from build123d import *

# Parameters (mm, degrees)
F0_W     = 101.6
F0_H     = 101.6
F1_DEPTH = 38.1
F3_DEPTH = 101.601
F5_DEPTH = 101.601
F6_R     = 5.08


with BuildPart() as f1:
    # F0 (on Top) → F1 (new body)
    with BuildSketch(Plane.XY):
        with Locations((4.577692, -1.507951)):
            Rectangle(F0_W, F0_H)
    extrude(amount=F1_DEPTH)

    # F2 (on face) → F3 (cut, through all)
    with BuildSketch(Plane.XZ.offset(52.307951)):
        Polygon((10.344626, 38.1), (-1.188108, 38.1), (-8.121741, 19.05), (17.278259, 19.05), align=None)
    extrude(amount=-F3_DEPTH, mode=Mode.SUBTRACT)

    # F4 (on face) → F5 (cut, through all)
    with BuildSketch(Plane(origin=(-46.222308, 0, 0), x_dir=(0, -1, 0), z_dir=(-1, 0, 0))):
        Polygon((7.274885, 38.1), (-4.257849, 38.1), (-11.191482, 19.05), (14.208518, 19.05), align=None)
    extrude(amount=-F5_DEPTH, mode=Mode.SUBTRACT)

    # F6
    f6_edges = [f1.edges().sort_by_distance(p)[0] for p in [
        (32.861159, -52.307951, 38.1),
        (-23.705208, -52.307951, 38.1),
        (-46.222308, -29.791418, 38.1),
        (-46.222308, 26.774949, 38.1),
        (55.377692, 26.774949, 38.1),
        (55.377692, -29.791418, 38.1),
        (-23.705208, 49.292049, 38.1),
        (32.861159, 49.292049, 38.1),
        (-46.222308, -52.307951, 19.05),
        (55.377692, -52.307951, 19.05),
        (-46.222308, 49.292049, 19.05),
        (55.377692, 49.292049, 19.05),
    ]]
    fillet(f6_edges, radius=F6_R)


solid = f1.part
Part model, mm, in its own coordinate system. A direction names the side the tool comes from. Coordinates: 2 decimals unless noted, no trailing zeros. Loops run counter-clockwise (first coordinate to the right, second up) from the corner with the lowest first, then second, coordinate; pieces in that order, holes last. Notation, with made-up numbers: (79, 59) - (135, 59) arc R27 ccw to (135, 92) - close; hole circle Ø3 at (77.5, 33). An arc over 180 degrees is marked (long way). Write each question's results on one line, items separated by ' | '. Start each with the question number.
Q1. Which spindle directions (+Z, -Z, +X, -X, +Y, -Y) get a long thin tool onto all of the face, cutting with end or side? Do faces 4 (the flat face through (-24.02, -10.79, 28.44)), 5 (the flat face through (30, 25, 38.1)). Say none if no direction does.
Q2. Probe line 1 along Z through (x, y) = (-1, 22); line 2 along Y through (x, z) = (20, 26.5); line 3 along X through (y, z) = (-16.5, 31). List the from-to ranges inside material, lowest first.
Q3. Two-plate mould, pull along Z, no slides. Class faces 1 (the flat face through (4, -1, 0)), 2 (the flat face through (13.86, -30.11, 28.44)), 3 (the cylindrical face through (-44.774, -50.78, 16.741)): +Z half, -Z half, draft (parallel to the pull), parting line (faces both ways), or undercut.
Q4. Slice it at D-D on z = 21. Give the cut face in (x, y).
Q5. Slice it at C-C on y = 34.5. Give the cut face in (x, z).
Q6. Slice it at A-A on z = 26.5. Give the cut face in (x, y), and give its area (3 significant figures).
Q7. Drop a flat-ended pin along its axis: pin 1 Ø5 at (x, y) = (1.5, 25) entering from +Z. Give the stop position or say it passes through.
Q8. Slice it at B-B on x = -32. Give the cut face in (y, z).
Answer:
1) face 4: +X, -X | face 5: +Z, +X, -X, +Y, -Y
2) line 1: z = 0 to 19.05 | line 2: y = -52.31 to -11.5, 8.48 to 49.29 | line 3: x = -46.22 to -3.77, 12.93 to 55.38
3) face 1: -Z half | face 2: undercut | face 3: draft
4) outline: (-46.22, -47.23) arc R5.08 ccw to (-41.14, -52.31) - (-7.41, -52.31) - (-7.41, -13.5) - (-46.22, -13.5) - close; (-46.22, 10.48) - (-7.41, 10.48) - (-7.41, 49.29) - (-41.14, 49.29) arc R5.08 ccw to (-46.22, 44.21) - close; (16.57, -52.31) - (50.3, -52.31) arc R5.08 ccw to (55.38, -47.23) - (55.38, -13.5) - (16.57, -13.5) - close; (16.57, 10.48) - (55.38, 10.48) - (55.38, 44.21) arc R5.08 ccw to (50.3, 49.29) - (16.57, 49.29) - close
5) outline: (-46.22, 0) - (55.38, 0) - (55.38, 33.02) arc R5.08 ccw to (50.3, 38.1) - (10.34, 38.1) - (17.28, 19.05) - (-8.12, 19.05) - (-1.19, 38.1) - (-41.14, 38.1) arc R5.08 ccw to (-46.22, 33.02) - close
6) outline: (-46.22, -47.23) arc R5.08 ccw to (-41.14, -52.31) - (-5.41, -52.31) - (-5.41, -11.5) - (-46.22, -11.5) - close; (-46.22, 8.48) - (-5.41, 8.48) - (-5.41, 49.29) - (-41.14, 49.29) arc R5.08 ccw to (-46.22, 44.21) - close; (14.57, -52.31) - (50.3, -52.31) arc R5.08 ccw to (55.38, -47.23) - (55.38, -11.5) - (14.57, -11.5) - close; (14.57, 8.48) - (55.38, 8.48) - (55.38, 44.21) arc R5.08 ccw to (50.3, 49.29) - (14.57, 49.29) - close | area: 6,640 mm2
7) pin 1: stops at z = 19.05
8) outline: (-52.31, 0) - (49.29, 0) - (49.29, 33.02) arc R5.08 ccw to (44.21, 38.1) - (4.26, 38.1) - (11.19, 19.05) - (-14.21, 19.05) - (-7.27, 38.1) - (-47.23, 38.1) arc R5.08 ccw to (-52.31, 33.02) - close
